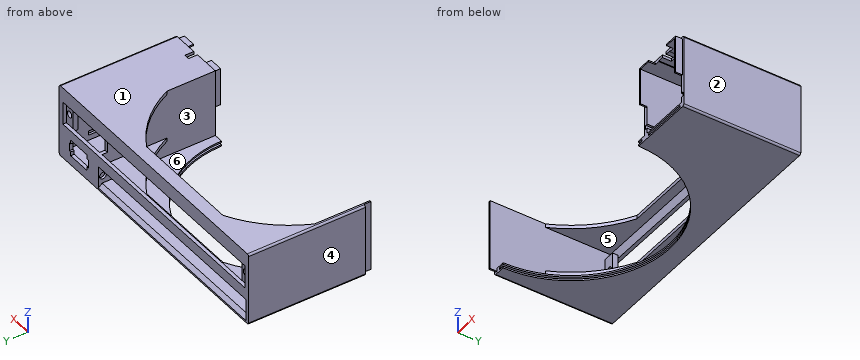
from build123d import *

# Parameters (mm, degrees)
ESQUISSE1_W              = 154.4
ESQUISSE1_H              = 40.8
BOSS_EXTRU_1_DEPTH       = 2
ESQUISSE2_W              = 154.4
ESQUISSE2_H              = 40.8
ESQUISSE2_W_2            = 120.4
ESQUISSE2_H_2            = 25.4
ESQUISSE2_H_3            = 8.4
ESQUISSE2_W_3            = 28
ESQUISSE2_H_4            = 35.8
BOSS_EXTRU_2_DEPTH       = 63.2
ENL_V_MAT_EXTRU_1_DEPTH  = 29.4
ESQUISSE8_W              = 9
ESQUISSE8_H              = 8.8
ENL_V_MAT_EXTRU_3_DEPTH  = 0.4
ESQUISSE9_W              = 3
ESQUISSE9_H              = 5
ENL_V_MAT_EXTRU_4_DEPTH  = 2.6
ESQUISSE10_W             = 1.2
ESQUISSE10_H             = 2.4
ENL_V_MAT_EXTRU_5_DEPTH  = 50.2
ESQUISSE12_W             = 0.8
ESQUISSE12_H             = 39.6
BOSS_EXTRU_3_DEPTH       = 3.8
ENL_V_MAT_EXTRU_6_REACH  = 71
ESQUISSE14_W             = 120.4
ESQUISSE14_H             = 8.4
ESQUISSE16_W             = 148.4
ESQUISSE16_H             = 12.9
ENL_V_MAT_EXTRU_8_DEPTH  = 2
ESQUISSE17_W             = 6.1
ESQUISSE17_H             = 16.9
ESQUISSE17_R             = 1.75
BOSS_EXTRU_5_DEPTH       = 3
ESQUISSE19_W             = 138.2
ESQUISSE19_H             = 12.9
ENL_V_MAT_EXTRU_10_DEPTH = 3
ESQUISSE20_R             = 1.9
ENL_V_MAT_EXTRU_11_DEPTH = 1.4
ESQUISSE21_R             = 1.9
ENL_V_MAT_EXTRU_12_DEPTH = 1.4
ENL_V_MAT_EXTRU_13_REACH = 42.8
ESQUISSE22_R             = 55.2
ENL_V_START              = -0.9
ESQUISSE23_R             = 58.2
ENL_V_MAT_EXTRU_14_DEPTH = 1.2
ENL_V_MAT_EXTRU_16_REACH = 71
ESQUISSE24_W             = 1.1
ESQUISSE24_H             = 4.7
ESQUISSE27_W             = 26
ESQUISSE27_H             = 3
ENL_V_MAT_EXTRU_17_DEPTH = 1.2
CONG_1_R                 = 1
CHANFREIN1_SIZE          = 2


with BuildPart() as part:
    # Esquisse1 → Boss.-Extru.1 (new body)
    with BuildSketch(Plane(origin=(0, 0, 0), x_dir=(1, 0, 0), z_dir=(0, 1, 0))):
        with Locations((77.2, 20.4)):
            Rectangle(ESQUISSE1_W, ESQUISSE1_H)
    extrude(amount=-BOSS_EXTRU_1_DEPTH)

    # Esquisse2 → Boss.-Extru.2 (add)
    with BuildSketch(Plane.XZ.offset(2)):
        with Locations((77.2, -20.4)):
            Rectangle(ESQUISSE2_W, ESQUISSE2_H)
        with Locations((62.2, -14.7)):
            Rectangle(ESQUISSE2_W_2, ESQUISSE2_H_2, mode=Mode.SUBTRACT)
        with Locations((62.2, -33.6)):
            Rectangle(ESQUISSE2_W_2, ESQUISSE2_H_3, mode=Mode.SUBTRACT)
        with Locations((138.4, -19.9)):
            Rectangle(ESQUISSE2_W_3, ESQUISSE2_H_4, mode=Mode.SUBTRACT)
    extrude(amount=BOSS_EXTRU_2_DEPTH)

    # Esquisse3 → Enlèv. mat.-Extru.1 (cut)
    with BuildSketch(Plane.XY):
        with BuildLine():
            Line((93.324909638, -7), (31.075090362, -7))
            ThreePointArc((31.075090362, -7), (13.955142399, -20.16186377), (2, -38.145240714))
            Line((2, -38.145240714), (2, -65.2))
            Line((2, -65.2), (122.4, -65.2))
            Line((122.4, -65.2), (122.4, -38.145240714))
            ThreePointArc((122.4, -38.145240714), (110.444857601, -20.16186377), (93.324909638, -7))
        make_face()
    extrude(amount=-ENL_V_MAT_EXTRU_1_DEPTH, mode=Mode.SUBTRACT)

    # Esquisse8 → Enlèv. mat.-Extru.3 (cut)
    with BuildSketch(Plane(origin=(0, 0, -2), x_dir=(-1, 0, 0), z_dir=(0, 0, -1))):
        with Locations((-138.4, -60.8)):
            Rectangle(ESQUISSE8_W, ESQUISSE8_H)
    extrude(amount=-ENL_V_MAT_EXTRU_3_DEPTH, mode=Mode.SUBTRACT)

    # Esquisse9 → Enlèv. mat.-Extru.4 (cut, through all)
    with BuildSketch(Plane(origin=(0, 0, -1.6), x_dir=(-1, 0, 0), z_dir=(0, 0, -1))):
        with Locations((-138.4, -62.7)):
            Rectangle(ESQUISSE9_W, ESQUISSE9_H)
    extrude(amount=-ENL_V_MAT_EXTRU_4_DEPTH, mode=Mode.SUBTRACT)

    # Esquisse10 → Enlèv. mat.-Extru.5 (cut)
    with BuildSketch(Plane.XZ.offset(65.2)):
        with Locations((153, -33.6)):
            Rectangle(ESQUISSE10_W, ESQUISSE10_H)
        with Locations((123.8, -33.6)):
            Rectangle(ESQUISSE10_W, ESQUISSE10_H)
    extrude(amount=-ENL_V_MAT_EXTRU_5_DEPTH, mode=Mode.SUBTRACT)

    # Esquisse12 → Boss.-Extru.3 (add)
    with BuildSketch(Plane.XZ.offset(65.2)):
        with Locations((1.6, -19.8)):
            Rectangle(ESQUISSE12_W, ESQUISSE12_H)
        Polygon((152.4, -2), (152.4, -22.2), (153.2, -22.2), (153.2, -1.2), (145.7, -1.2), (145.7, -2), align=None)
        Polygon((131.1, -2), (131.1, -1.2), (123.6, -1.2), (123.6, -22.2), (124.4, -22.2), (124.4, -2), align=None)
    extrude(amount=BOSS_EXTRU_3_DEPTH)

    # Esquisse14 → Enlèv. mat.-Extru.6 (cut, up to next)
    with BuildSketch(Plane(origin=(0, 0, 0), x_dir=(1, 0, 0), z_dir=(0, 1, 0)), mode=Mode.PRIVATE) as enl_v_mat_extru_6_sk1:
        with Locations((62.2, 33.6)):
            Rectangle(ESQUISSE14_W, ESQUISSE14_H)
    enl_v_mat_extru_6_tool1 = extrude(enl_v_mat_extru_6_sk1.sketch, amount=-ENL_V_MAT_EXTRU_6_REACH, mode=Mode.PRIVATE) & part.part
    add(enl_v_mat_extru_6_tool1.solids().sort_by_distance((62.2, 0, -33.6))[0], mode=Mode.SUBTRACT)

    # Esquisse16 → Enlèv. mat.-Extru.8 (cut)
    with BuildSketch(Plane(origin=(0, 0, 0), x_dir=(1, 0, 0), z_dir=(0, 1, 0))):
        with Locations((77.2, 14.7)):
            Rectangle(ESQUISSE16_W, ESQUISSE16_H)
    extrude(amount=-ENL_V_MAT_EXTRU_8_DEPTH, mode=Mode.SUBTRACT)

    # Esquisse17 → Boss.-Extru.5 (add)
    with BuildSketch(Plane.XZ.offset(2)):
        with Locations((5.05, -14.7)):
            Rectangle(ESQUISSE17_W, ESQUISSE17_H)
        with Locations((5.5, -14.7)):
            Circle(ESQUISSE17_R, mode=Mode.SUBTRACT)
        with Locations((149.35, -14.7)):
            Rectangle(ESQUISSE17_W, ESQUISSE17_H)
        with Locations((148.9, -14.7)):
            Circle(ESQUISSE17_R, mode=Mode.SUBTRACT)
    extrude(amount=BOSS_EXTRU_5_DEPTH)

    # Esquisse19 → Enlèv. mat.-Extru.10 (cut)
    with BuildSketch(Plane(origin=(0, -2, 0), x_dir=(1, 0, 0), z_dir=(0, 1, 0))):
        with Locations((77.2, 14.7)):
            Rectangle(ESQUISSE19_W, ESQUISSE19_H)
    extrude(amount=-ENL_V_MAT_EXTRU_10_DEPTH, mode=Mode.SUBTRACT)

    # Esquisse20 → Enlèv. mat.-Extru.11 (cut)
    with BuildSketch(Plane.ZY.offset(-122.4)):
        with Locations((-33.6, -2.5)):
            Circle(ESQUISSE20_R)
    extrude(amount=-ENL_V_MAT_EXTRU_11_DEPTH, mode=Mode.SUBTRACT)

    # Esquisse21 → Enlèv. mat.-Extru.12 (cut)
    with BuildSketch(Plane(origin=(2, 0, 0), x_dir=(0, 0, -1), z_dir=(1, 0, 0))):
        with Locations((33.6, -2.5)):
            Circle(ESQUISSE21_R)
    extrude(amount=-ENL_V_MAT_EXTRU_12_DEPTH, mode=Mode.SUBTRACT)

    # Esquisse22 → Enlèv. mat.-Extru.13 (cut, up to next)
    with BuildSketch(Plane(origin=(0, 0, -40.8), x_dir=(-1, 0, 0), z_dir=(0, 0, -1)), mode=Mode.PRIVATE) as enl_v_mat_extru_13_sk1:
        with Locations((-62.2, -65.2)):
            Circle(ESQUISSE22_R)
    enl_v_mat_extru_13_tool1 = extrude(enl_v_mat_extru_13_sk1.sketch, amount=-ENL_V_MAT_EXTRU_13_REACH, mode=Mode.PRIVATE) & part.part
    add(enl_v_mat_extru_13_tool1.solids().sort_by_distance((62.2, -65.2, -40.8))[0], mode=Mode.SUBTRACT)

    # Esquisse23 → Enlèv. mat.-Extru.14 (cut)
    with BuildSketch(Plane(origin=(0, 0, -40.8), x_dir=(-1, 0, 0), z_dir=(0, 0, -1)).offset(ENL_V_START)):
        with Locations((-62.2, -65.2)):
            Circle(ESQUISSE23_R)
    extrude(amount=-ENL_V_MAT_EXTRU_14_DEPTH, mode=Mode.SUBTRACT)

    # Esquisse24 → Enlèv. mat.-Extru.16 (cut, up to next)
    with BuildSketch(Plane(origin=(0, 0, 0), x_dir=(1, 0, 0), z_dir=(0, 1, 0)), mode=Mode.PRIVATE) as enl_v_mat_extru_16_sk1:
        Polygon((131.7, 35.525), (145.1, 35.525), (145.1, 26.425), (131.7, 26.425), (131.7, 28.625), (130.6, 28.625), (130.6, 33.325), (131.7, 33.325), align=None)
    enl_v_mat_extru_16_tool1 = extrude(enl_v_mat_extru_16_sk1.sketch, amount=-ENL_V_MAT_EXTRU_16_REACH, mode=Mode.PRIVATE) & part.part
    add(enl_v_mat_extru_16_tool1.solids().sort_by_distance((138.105118, 0, -30.975))[0], mode=Mode.SUBTRACT)
    # Esquisse24 → Enlèv. mat.-Extru.16 (cut, up to next)
    with BuildSketch(Plane(origin=(0, 0, 0), x_dir=(1, 0, 0), z_dir=(0, 1, 0)), mode=Mode.PRIVATE) as enl_v_mat_extru_16_sk2:
        with Locations((145.65, 30.975)):
            Rectangle(ESQUISSE24_W, ESQUISSE24_H)
    enl_v_mat_extru_16_tool2 = extrude(enl_v_mat_extru_16_sk2.sketch, amount=-ENL_V_MAT_EXTRU_16_REACH, mode=Mode.PRIVATE) & part.part
    add(enl_v_mat_extru_16_tool2.solids().sort_by_distance((145.65, 0, -30.975))[0], mode=Mode.SUBTRACT)

    # Esquisse27 → Enlèv. mat.-Extru.17 (cut)
    with BuildSketch(Plane.XY.offset(-37.8).offset(ENL_V_START)):
        with Locations((138.4, -63.7)):
            Rectangle(ESQUISSE27_W, ESQUISSE27_H)
    extrude(amount=-ENL_V_MAT_EXTRU_17_DEPTH, mode=Mode.SUBTRACT)

    # Congé1
    cong_1_edges = [part.edges().sort_by_distance(p)[0] for p in [
        (0, -32.6, -40.8),
        (154.4, -32.6, -40.8),
        (154.4, -32.6, 0),
        (0, -32.6, 0),
    ]]
    fillet(cong_1_edges, radius=CONG_1_R)

    # Chanfrein1
    chanfrein1_edges = [part.edges().sort_by_distance(p)[0] for p in [
        (62.2, 0, -29.4),
        (62.2, 0, -37.8),
    ]]
    chamfer(chanfrein1_edges, length=CHANFREIN1_SIZE)


solid = part.part
Read the model definition and answer for the solid it produces. Units are mm, in the model's axes. Face numbers are marked on the shaded views. A direction names the side the tool comes from. Give positions to 0.01 mm unless a question says otherwise; leave off trailing zeros. Write each loop counter-clockwise with the first axis right and the second up, starting at its lowest first coordinate (ties: lowest second). Pieces come first, ordered by that corner, then holes. Notation, with made-up numbers: (-31, 73.25) - (0, 73.25) arc R18 cw to (0, 81.25) - close; hole circle Ø9 at (81.25, 24). An arc over 180 degrees is marked (long way). Use CSV: the item, a comma, the result in double quotes. Start each with the question number.
(1) Find section B-B (z = -18). Give the vertices of the cut face in (x, y).
(2) Determine the mould class of the marked faces 1, 2 and 3 for opening direction X: +X half, -X half, draft (parallel to the pull), parting line (faces both ways), or undercut.
(3) Find section D-D (y = -53). Count the separate pieces of the cut face and the enclosed holes in it, plus the area to 3 significant figures.
(4) Given P1, Ø3, axis at y = -67, z = -16, coming from the +X side; P2, Ø10, axis at x = 132.5, z = -18.5, coming from the -Y side; P3, Ø0.9, axis at y = -67, z = -1.5, coming from the -X side, each flat-ended and moving along its own axis, determine where each tip first touches the part or whether it passes through.
(5) For the marked faces 4, 5 and 6, determine the directions among +Z, -Z, +X, -X, +Y, -Y from which every point of the face is accessible in a straight line to the end or side of a thin tool.
(6) Find section A-A (x = 148.9). Give the vertices of the cut face in (y, z).
(7) Find section C-C (x = 62.2). Give the vertices of the cut face in (y, z), plus the area to 3 significant figures.
(8) Consider line 1 along X through (y, z) = (-4, -37); line 2 along X through (y, z) = (-65.5, -13); line 3 along Z through (x, y) = (148.9, -3.2). Determine where each line is inside the solid, lowest interval first.
Findings below:
1,outline,"(0, -65.2) - (1.2, -65.2) - (1.2, -69) - (2, -69) - (2, -5) - (8.1, -5) - (8.1, -2) - (3, -2) - (3, 0) - (0, 0) - close; (122.4, -65.2) - (123.6, -65.2) - (123.6, -69) - (124.4, -69) - (124.4, -5) - (122.4, -5) - close; (146.3, -5) - (152.4, -5) - (152.4, -69) - (153.2, -69) - (153.2, -65.2) - (154.4, -65.2) - (154.4, 0) - (151.4, 0) - (151.4, -2) - (146.3, -2) - close"
2,face 1,"draft"
2,face 2,"+X half"
2,face 3,"undercut"
3,separate pieces,"2"
3,enclosed holes,"1"
3,area,"409 mm2"
4,P1,"x = 153.2"
4,P2,"y = -2"
4,P3,"x = 1.2"
5,face 4,"+Z, -Z, -X, +Y, -Y"
5,face 5,"-Y"
5,face 6,"+Y, -Y"
6,outline,"(-69, -2) - (-2, -2) - (-2, -6.25) - (-5, -6.25) - (-5, -12.95) - (-2, -12.95) - (-2, -8.25) - (0, -8.25) - (0, 0) - (-65.2, 0) - (-65.2, -1.2) - (-69, -1.2) - close; (-65.2, -40.8) - (0, -40.8) - (0, -21.15) - (-2, -21.15) - (-2, -16.45) - (-5, -16.45) - (-5, -23.15) - (-2, -23.15) - (-2, -37.8) - (-65.2, -37.8) - (-65.2, -38.7) - (-62.2, -38.7) - (-62.2, -39.9) - (-65.2, -39.9) - close"
7,outline,"(-10, -40.8) - (0, -40.8) - (0, -39.8) - (-2, -37.8) - (-10, -37.8) - (-10, -38.7) - (-7, -38.7) - (-7, -39.9) - (-10, -39.9) - close; (-7, -29.4) - (-2, -29.4) - (0, -27.4) - (0, -21.15) - (-2, -21.15) - (-2, -27.4) - (-7, -27.4) - close; (-7, -2) - (-2, -2) - (-2, -8.25) - (0, -8.25) - (0, 0) - (-7, 0) - close"
7,area,"75.4 mm2"
8,line 1,"0 to 2, 122.4 to 124.4, 152.4 to 154.4"
8,line 2,"1.2 to 2, 123.6 to 124.4, 152.4 to 153.2"
8,line 3,"-40.8 to -37.8, -23.15 to -16.45, -12.95 to -6.25, -2 to 0"
